Source: CAD feature listing. Evaluate the final solid. Frame: model axes, mm. Give positions to 0.01 mm unless a question says otherwise; leave off trailing zeros. Loops run counter-clockwise (first coordinate to the right, second up) from the corner with the lowest first, then second, coordinate; pieces in that order, holes last. Notation, with made-up numbers: M -30,75 L -10,75 A29 ccw -10,105 Z; hole C -15,27 d6. An arc over 180 degrees is marked long. Write item = value, one per line.
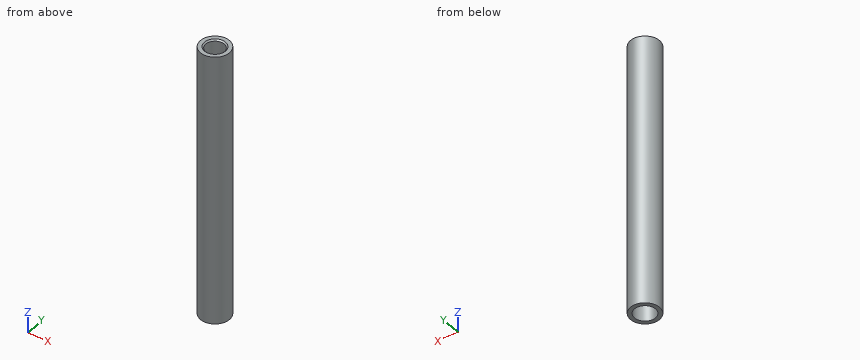
from build123d import *

# Parameters (mm, degrees)
SZKIC1_R                    = 11
SZKIC1_R_2                  = 7
DODANIE_WYCI_GNI_CIE1_DEPTH = 102.5
SZKIC2_R                    = 8
WYTNIJ_WYCI_GNI_CIE1_DEPTH  = 50
SFAZOWANIE1_SIZE            = 1


with BuildPart() as part:
    # Szkic1 → Dodanie-wyciągnięcie1 (new, symmetric)
    with BuildSketch(Plane.XY):
        with Locations(Location((0, 0, 0), (0, 0, 180))):
            Circle(SZKIC1_R)
        with Locations(Location((0, 0, 0), (0, 0, 180))):
            Circle(SZKIC1_R_2, mode=Mode.SUBTRACT)
    extrude(amount=DODANIE_WYCI_GNI_CIE1_DEPTH, both=True)

    # Szkic2 → Wytnij-wyciągnięcie1 (cut)
    with BuildSketch(Plane(origin=(0, 0, -102.5), x_dir=(-1, 0, 0), z_dir=(0, 0, -1))):
        Circle(SZKIC2_R)
    extrude(amount=-WYTNIJ_WYCI_GNI_CIE1_DEPTH, mode=Mode.SUBTRACT)

    # Sfazowanie1
    sfazowanie1_edges = [part.edges().sort_by_distance(p)[0] for p in [
        (7, 0, 102.5),
    ]]
    chamfer(sfazowanie1_edges, length=SFAZOWANIE1_SIZE)


solid = part.part
1. Material intervals for probe 1 along Y at (x, z) = (0, 56); probe 2 along Y at (x, z) = (-6, 55); probe 3 along Y at (x, z) = (-9.5, 43), sorted ascending. Write a range as from..to.
Derived:
probe_1 = -11..-7, 7..11
probe_2 = -9.22..-3.61, 3.61..9.22
probe_3 = -5.55..5.55
2. Cut plane D-D, the plane z = -82. Return the cut outline in (x, y), then the cut area to 3 significant figures.
Derived:
outline = C 0,0 d22; hole C 0,0 d16
area = 179 mm²
3. Cut plane C-C, the plane z = -16. Return the cut outline in (x, y).
Derived:
outline = C 0,0 d22; hole C 0,0 d14
4. First-contact query: pin 1 Ø4 at (x, z) = (-4, 79) entering from -Y; pin 2 Ø3 at (x, z) = (-7, -10) entering from -Y; pin 3 Ø3 at (x, y) = (-3, 3.5) entering from -Z; pin 4 Ø5 at (y, z) = (3, 26) entering from +X. Flat tips, straight axial feed; report the tip coordinate or a pass-through.
Derived:
pin_1 = -10.82
pin_2 = -9.53
pin_3 = through
pin_4 = 10.99
5. Cut plane A-A, the plane x = 0. Return the cut outline in (y, z).
Derived:
outline = M -11,-102.5 L -8,-102.5 L -8,-52.5 L -7,-52.5 L -7,101.5 L -8,102.5 L -11,102.5 Z; M 7,-52.5 L 8,-52.5 L 8,-102.5 L 11,-102.5 L 11,102.5 L 8,102.5 L 7,101.5 Z
